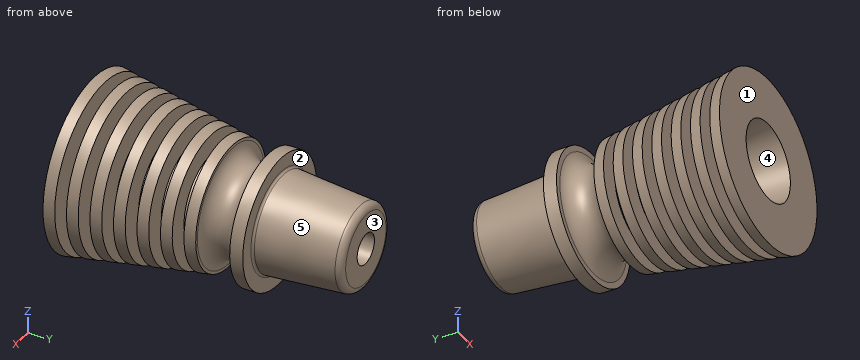
from build123d import *

# Parameters (mm, degrees)
SKETCH5_R          = 1.6383
CUT_EXTRUDE1_DEPTH = 30.2608
FILLET1_R          = 0.762
FILLET2_R          = 0.254


with BuildPart() as part:
    # Sketch1 → Revolve1 (revolve)
    with BuildSketch(Plane.XY, mode=Mode.PRIVATE) as revolve1_sk:
        Polygon((4.571997254, 14.859), (6.235697254, 0), (4.191, 0), (2.5273, 14.859), align=None)
    revolve(revolve1_sk.sketch.rotate(Axis((0, 0, 0), (0, 1, 0)), 90), axis=Axis((0, 0, 0), (0, 1, 0)))  # turned: the seam where the file's is

    # Sketch2 → Revolve2 (revolve)
    with BuildSketch(Plane.XY, mode=Mode.PRIVATE) as revolve2_sk:
        Polygon((6.235697254, 0), (9.2329, 0), (9.035561538, 1.143), (6.107720331, 1.143), align=None)
        Polygon((4.571997254, 14.859), (4.699974177, 13.716), (6.864838462, 13.716), (6.6675, 14.859), align=None)
        Polygon((5.979743408, 2.286), (8.838223077, 2.286), (8.640884615, 3.429), (5.851766485, 3.429), align=None)
        Polygon((5.723789562, 4.572), (8.443546154, 4.572), (8.246207692, 5.715), (5.595812639, 5.715), align=None)
        Polygon((5.467835716, 6.858), (8.048869231, 6.858), (7.851530769, 8.001), (5.339858793, 8.001), align=None)
        Polygon((5.21188187, 9.144), (7.654192308, 9.144), (7.456853846, 10.287), (5.083904947, 10.287), align=None)
        Polygon((4.955928023, 11.43), (7.259515385, 11.43), (7.062176923, 12.573), (4.8279511, 12.573), align=None)
    revolve(revolve2_sk.sketch.rotate(Axis((0, 0, 0), (0, 1, 0)), 90), axis=Axis((0, 0, 0), (0, 1, 0)))  # turned: the seam where the file's is

    # Sketch3 → Revolve3 (revolve)
    with BuildSketch(Plane.XY, mode=Mode.PRIVATE) as revolve3_sk:
        with BuildLine():
            Line((6.35, 14.859), (0, 14.859))
            Line((0, 14.859), (0, 20.066))
            Line((0, 20.066), (6.985, 20.066))
            Line((6.985, 20.066), (6.985, 18.669))
            Line((6.985, 18.669), (6.35, 18.669))
            ThreePointArc((6.35, 18.669), (4.6863, 16.764), (6.35, 14.859))
        make_face()
    revolve(revolve3_sk.sketch.rotate(Axis((0, 0, 0), (0, 1, 0)), 90), axis=Axis((0, 0, 0), (0, 1, 0)))  # turned: the seam where the file's is

    # Sketch4 → Revolve4 (revolve)
    with BuildSketch(Plane.XY, mode=Mode.PRIVATE) as revolve4_sk:
        Polygon((5.2197, 20.066), (0, 20.066), (0, 29.2608), (4.5212, 29.2608), align=None)
    revolve(revolve4_sk.sketch.rotate(Axis((0, 0, 0), (0, 1, 0)), 90), axis=Axis((0, 0, 0), (0, 1, 0)))  # turned: the seam where the file's is

    # Sketch5 → Cut-Extrude1 (cut, through all)
    with BuildSketch(Plane(origin=(0, 29.2608, 0), x_dir=(1, 0, 0), z_dir=(0, 1, 0))):
        with Locations(Location((0, 0, 0), (0, 0, 270))):  # turned: the seam where the file's is
            Circle(SKETCH5_R)
    extrude(amount=-CUT_EXTRUDE1_DEPTH, mode=Mode.SUBTRACT)

    # Fillet1
    fillet1_edges = [part.edges().sort_by_distance(p)[0] for p in [
        (0, 29.2608, 4.5212),
    ]]
    fillet(fillet1_edges, radius=FILLET1_R)

    # Fillet2
    fillet2_edges = [part.edges().sort_by_distance(p)[0] for p in [
        (0, 20.066, 5.2197),
    ]]
    fillet(fillet2_edges, radius=FILLET2_R)


solid = part.part
The model under review builds one solid part; all positions refer to its coordinate system, in mm. Face numbers are marked on the shaded views. A direction names the side the tool comes from. Give positions to 0.01 mm unless a question says otherwise; leave off trailing zeros. Write each loop counter-clockwise with the first axis right and the second up, starting at its lowest first coordinate (ties: lowest second). Pieces come first, ordered by that corner, then holes. Notation, with made-up numbers: M 38.25,26.25 L 88.25,26.25 A19 cw 88.25,62.25 Z; hole C 50,74 d11. An arc over 180 degrees is marked long. One line per question, with ' | ' between items. Start each with the question number.
Item 1: Wall thickness on line 1 (X direction, y = 25.25, z = 0); line 2 (X direction, y = 21.75, z = 0); line 3 (Y direction, x = 4.75, z = -2.5): over which ranges is each line inside the solid? List them lowest first. Write a range as from..to.
Item 2: We need section B-B on y = 26. Write out the cut boundary in (x, z), plus the area to 3 significant figures.
Item 3: For pin 1 (4 mm diameter, centred on x = -2, z = -1.5, fed in from -Y); pin 2 (2 mm diameter, centred on y = 15, z = -0.5, fed in from +X); pin 3 (5 mm diameter, centred on x = 3.5, y = 25, fed in from -Z); pin 4 (3 mm diameter, centred on x = 0, z = 0, fed in from +Y), all flat-tipped, find the tip position at first contact; note any pin that passes through.
Item 4: For the marked faces 1 and 2, list the 3-axis set-ups (+Z, -Z, +X, -X, +Y, -Y) from which the entire face can be reached by the end or side of a thin tool; tool diameter is ignored.
Item 5: We need section A-A on y = 22.5. Write out the cut boundary in (x, z).
Item 6: Draft analysis for pull direction Z (two halves, no side actions). For the marked faces 3, 4 and 5, state which applies: released by +Z, released by -Z, zero draft, split by the parting line, or undercut.
Results found:
1) line 1: x = -4.83..-1.64, 1.64..4.83 | line 2: x = -5.09..-1.64, 1.64..5.09 | line 3: y = 0..8, 9.14..10.29, 11.43..12.57, 13.72..15.3, 18.23..20.08
2) outline: C 0,0 d9.54; hole C 0,0 d3.28 | area: 63.0 mm2
3) pin 1: stops at y = 0 | pin 2: stops at x = 6.81 | pin 3: stops at z = -4.77 | pin 4: passes through
4) face 1: +Z, -Z, +X, -X, -Y | face 2: +Y
5) outline: C 0,0 d10.07; hole C 0,0 d3.28
6) face 3: zero draft | face 4: undercut | face 5: split by the parting line
